from build123d import *

# Parameters (mm, degrees)
SKETCH1_W               = 26
SKETCH1_H               = 15
SKETCH1_R               = 2
BOSS_EXTRUDE1_DEPTH     = 1
FILLET1_R               = 1
SKETCH3_R               = 1.5
BOSS_EXTRUDE2_DEPTH     = 26
BOSS_EXTRUDE3_REACH     = 32.083
SKETCH6_W               = 26
SKETCH6_H               = 1
CUT_EXTRUDE1_DEPTH      = 31.083217913
CUT_EXTRUDE1_DEPTH_BACK = 31.083217913
SKETCH8_W               = 6.5
SKETCH8_H               = 3.1


with BuildPart() as part:
    # Sketch1 → Boss-Extrude1 (new body)
    with BuildSketch(Plane.XY):
        with Locations((13, 7.5)):
            Rectangle(SKETCH1_W, SKETCH1_H)
        with Locations((6, 7)):
            Circle(SKETCH1_R, mode=Mode.SUBTRACT)
        with Locations((20, 7)):
            Circle(SKETCH1_R, mode=Mode.SUBTRACT)
    extrude(amount=BOSS_EXTRUDE1_DEPTH)

    # Fillet1
    fillet1_edges = [part.edges().sort_by_distance(p)[0] for p in [
        (0, 15, 0.5),
        (26, 15, 0.5),
    ]]
    fillet(fillet1_edges, radius=FILLET1_R)


with BuildPart() as body_2:
    # Sketch3 → Boss-Extrude2 (new body)
    with BuildSketch(Plane(origin=(0, 0, 0), x_dir=(0, 0, -1), z_dir=(1, 0, 0))):
        with Locations(Location((-0.5, -1.6, 0), (0, 0, 180))):
            Circle(SKETCH3_R)
    extrude(amount=BOSS_EXTRUDE2_DEPTH)

    # Sketch6 → Boss-Extrude3 (add, up to next)
    with BuildSketch(Plane.XZ, mode=Mode.PRIVATE) as boss_extrude3_sk1:
        with Locations((13, 0.5)):
            Rectangle(SKETCH6_W, SKETCH6_H)
    boss_extrude3_tool1 = extrude(boss_extrude3_sk1.sketch, amount=BOSS_EXTRUDE3_REACH, mode=Mode.PRIVATE) - body_2.part

    add(part.part)  # Boss-Extrude3 merges part
    add(boss_extrude3_tool1.solids().sort_by_distance((13, 0, 0.5))[0])

    # Sketch8 → Cut-Extrude1 (cut, two sides: drawn at the far end of the back side and taken through both)
    with BuildSketch(Plane.XY.offset(-CUT_EXTRUDE1_DEPTH_BACK)):
        with Locations((3.25, -1.55)):
            Rectangle(SKETCH8_W, SKETCH8_H)
        with Locations((16.25, -1.55)):
            Rectangle(SKETCH8_W, SKETCH8_H)
    extrude(amount=CUT_EXTRUDE1_DEPTH + CUT_EXTRUDE1_DEPTH_BACK, mode=Mode.SUBTRACT)


solid = body_2.part
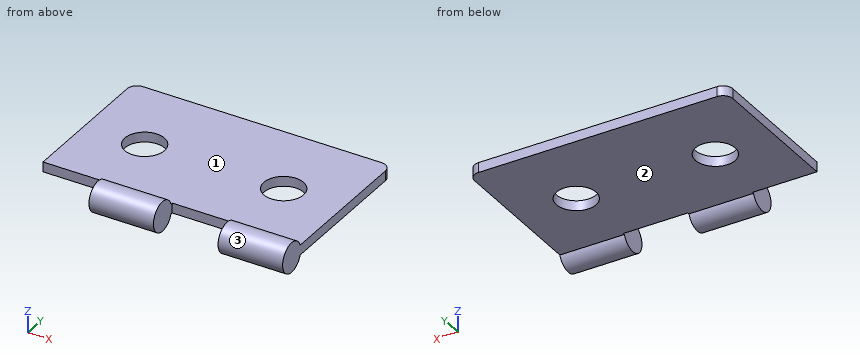
Geometry: final body of the model. Coordinates: model frame, mm. Face numbers are marked on the shaded views. A direction names the side the tool comes from. Give positions to 0.01 mm unless a question says otherwise; leave off trailing zeros. Write each loop counter-clockwise with the first axis right and the second up, starting at its lowest first coordinate (ties: lowest second). Pieces come first, ordered by that corner, then holes. Notation, with made-up numbers: M 42,7 L 75,7 A16 ccw 75,36 Z; hole C -40,-29 d10. An arc over 180 degrees is marked long. Answer in a Markdown table with one row per item. Add a question column.
(1) Reachability of the marked faces 1, 2 and 3 from +Z, -Z, +X, -X, +Y, -Y: full face, straight path, thin tool, end or side. Return the list, or none.
(2) Section C-C on z = 0.5. Return loops of the section in (x, y), and give its area (3 significant figures).
(3) Section A-A on y = -1.6. Return loops of the section in (x, z), and give its area (3 significant figures).
(4) Ray query, line 1 (Y direction, x = 6, z = 0.75); line 2 (Y direction, x = 20, z = 0.5); line 3 (Z direction, x = 8.75, y = 2.75). Return the intervals inside material, ascending.
(5) Section D-D on x = 16.25. Return loops of the section in (y, z).
(6) First-contact query: pin 1 (6 mm diameter, centred on x = 15, y = 12.5, fed in from -Z); pin 2 (1.5 mm diameter, centred on y = -2, z = 0, fed in from -X); pin 3 (5 mm diameter, centred on x = 5.5, y = 8.5, fed in from +Z). Flat tips, straight axial feed; report the tip coordinate or a pass-through.
(7) Section B-B on x = 20. Return loops of the section in (y, z).
Result set:
| question | item | result |
|---|---|---|
| 1 | face 1 | +Z, +X, -X, +Y |
| 1 | face 2 | -Z, +X, -X, +Y |
| 1 | face 3 | +X, -X |
| 2 | outline | M 0,0 L 6.5,0 L 6.5,-3.1 L 13,-3.1 L 13,0 L 19.5,0 L 19.5,-3.1 L 26,-3.1 L 26,14 A1 ccw 25,15 L 1,15 A1 ccw 0,14 Z; hole C 6,7 d4; hole C 20,7 d4 |
| 2 | area | 405 mm^2 |
| 3 | outline | M 6.5,-1 L 13,-1 L 13,2 L 6.5,2 Z; M 19.5,-1 L 26,-1 L 26,2 L 19.5,2 Z |
| 3 | area | 39.0 mm^2 |
| 4 | line 1 | y = 0 to 5, 9 to 15 |
| 4 | line 2 | y = -3.1 to 5, 9 to 15 |
| 4 | line 3 | z = 0 to 1 |
| 5 | outline | M 0,0 L 15,0 L 15,1 L 0,1 Z |
| 6 | pin 1 | stops at z = 0 |
| 6 | pin 2 | stops at x = 6.5 |
| 6 | pin 3 | stops at z = 1 |
| 7 | outline | M -0.19,0 L 5,0 L 5,1 L -0.19,1 A1.5 ccw long Z; M 9,0 L 15,0 L 15,1 L 9,1 Z |
